Design review of the part built by this model. Coordinates are the model's own, in mm. Give positions to 0.01 mm unless a question says otherwise; leave off trailing zeros. Write each loop counter-clockwise with the first axis right and the second up, starting at its lowest first coordinate (ties: lowest second). Pieces come first, ordered by that corner, then holes. Notation, with made-up numbers: (-31.5, -38) - (-6.5, -38) arc R25 ccw to (-6.5, -12) - close; hole circle Ø1 at (-4.5, 74). An arc over 180 degrees is marked (long way). Write each question's results on one line, items separated by ' | '. Start each with the question number.
from build123d import *

# Parameters (mm, degrees)
SKETCH1_R    = 5
SKETCH1_R_2  = 2.65
SPACER_DEPTH = 8
FILLET1_R    = 0.5


with BuildPart() as part:
    # Sketch1 → spacer (new body)
    with BuildSketch(Plane.XY):
        Circle(SKETCH1_R)
        Circle(SKETCH1_R_2, mode=Mode.SUBTRACT)
    extrude(amount=SPACER_DEPTH)

    # Fillet1
    fillet1_edges = [part.edges().sort_by_distance(p)[0] for p in [
        (-5, 0, 0),
        (-5, 0, 8),
        (-2.65, 0, 0),
        (-2.65, 0, 8),
    ]]
    fillet(fillet1_edges, radius=FILLET1_R)


solid = part.part
Q1. The part is to be moulded in two halves that separate along Y. For faces 1 (the face through (-1.08, -4.88, 3.95)), 2 (the face through (2, -3, 0)), 3 (the face through (2.45, -1.01, 3.95)), say which applies: +Y half, -Y half, draft (parallel to the pull), parting line (faces both ways), or undercut.
Q2. Insertion check: P1, Ø1.5, axis at y = 3.5, z = 6.5, coming from the -X side; P2, Ø1, axis at x = 1.5, z = 4.5, coming from the -Y side; P3, Ø1.5, axis at x = -2, y = 1, coming from the +Z side; P4, Ø4, axis at x = 0, y = 0, coming from the +Z side. Each pin has a flat end and moves straight along its axis. Give the tip position at first contact, or say it passes through.
Q3. Add section A-A on y = 0. State the section outline as (x, z) points.
Q4. For line 1 along Y through (x, z) = (0, 4.5); line 2 along X through (y, z) = (1.25, 6.5); line 3 along Y through (x, z) = (2, 1), list the stretches that pass through material, from the lowest coordinate up. Write a range as [from, to].
Q5. Add section C-C on z = 6.25. State the section outline as (x, y) points.
Result:
1) face 1: parting line | face 2: draft | face 3: undercut
2) P1: stops at x = -4.18 | P2: stops at y = -4.9 | P3: stops at z = 7.97 | P4: passes through
3) outline: (-5, 0.5) arc R0.5 ccw to (-4.5, 0) - (-3.15, 0) arc R0.5 ccw to (-2.65, 0.5) - (-2.65, 7.5) arc R0.5 ccw to (-3.15, 8) - (-4.5, 8) arc R0.5 ccw to (-5, 7.5) - close; (2.65, 0.5) arc R0.5 ccw to (3.15, 0) - (4.5, 0) arc R0.5 ccw to (5, 0.5) - (5, 7.5) arc R0.5 ccw to (4.5, 8) - (3.15, 8) arc R0.5 ccw to (2.65, 7.5) - close
4) line 1: y = [-5, -2.65], [2.65, 5] | line 2: x = [-4.84, -2.34], [2.34, 4.84] | line 3: y = [-4.58, -1.74], [1.74, 4.58]
5) outline: circle Ø10 at (0, 0); hole circle Ø5.3 at (0, 0)
